For this review, take the finished solid that the model builds, in its own axes (mm). A direction names the side the tool comes from. Round coordinates to 2 decimals unless told otherwise and drop trailing zeros. Write each loop counter-clockwise with the first axis right and the second up, starting at its lowest first coordinate (ties: lowest second). Pieces come first, ordered by that corner, then holes. Notation, with made-up numbers: M 84,53 L 115,53 A12 cw 115,62 Z; hole C 25.5,59 d1. An arc over 180 degrees is marked long. Use one line per item in the form item = value. Start each with the question number.
Item 1: Add section C-C (z = 26). State the section outline as (x, y) points.
Item 2: Draft analysis for pull direction X (two halves, no side actions). For faces 1 (the flat face through (-10, 0, 25)), 2 (the flat face through (19.233, -17, 25)), 3 (the flat face through (-5, -92, 25)), state which applies: released by +X, released by -X, zero draft, split by the parting line, or undercut.
Item 3: Add section D-D (x = -22). State the section outline as (y, z) points, and give its area (3 significant figures).
Item 4: Add section B-B (x = 11). State the section outline as (y, z) points.
Item 5: Add section A-A (y = -18). State the section outline as (x, z) points, and give its area (3 significant figures).
Item 6: For P1, Ø2, axis at y = -21, z = 35, coming from the -X side; P2, Ø10, axis at y = -53.5, z = 5, coming from the +X side; P3, Ø4.5, axis at x = 31, y = -69, coming from the +Z side, all flat-tipped, find the tip position at first contact; note any pin that passes through.
Item 7: For faces 4 (the cylindrical face through (13.724, -86.113, 27.185)), 5 (the flat face through (5, -92, 25)), 6 (the flat face through (-5, -10, 25)), 7 (the flat face through (-19.233, -16, 25)), 8 (the flat face through (7, -93, 27)), list the 3-axis set-ups (+Z, -Z, +X, -X, +Y, -Y) from which the entire face can be reached by the end or side of a thin tool; tool diameter is ignored.
Item 8: For line 1 (X direction, y = -8, z = 37); line 2 (Y direction, x = 0, z = 28); line 3 (X direction, y = -20.5, z = 43.5), list the stretches that pass through material, from the lowest coordinate up. Write a range as [from, to].
from build123d import *

# Parameters (mm, degrees)
F1_DEPTH = 50
F2_DEPTH = 5


# Not quite as in the source:
# - a feature of the source that left no trace in its solid (it failed there, or was rolled back) is left out


with BuildPart() as f1:
    # F0 (on Top) → F1 (new body)
    with BuildSketch(Plane.XY):
        with BuildLine():
            Line((-19.2333690145, -5), (-19.2333690145, -27.8079588042))
            ThreePointArc((-19.2333690145, -27.8079588042), (-36.7344496958, -67.5385811362), (-5, -97.1651718683))
            Line((-5, -97.1651718683), (-5, -87.041634566))
            ThreePointArc((-5, -87.041634566), (-17.5890590993, -38.8605818434), (27.5, -60))
            ThreePointArc((27.5, -60), (25.4982682633, -70.2999182314), (19.7844861402, -79.1003693203))
            ThreePointArc((19.7844861402, -79.1003693203), (13.0128248945, -84.2263573049), (5, -87.041634566))
            Line((5, -87.041634566), (5, -97.1651718683))
            ThreePointArc((5, -97.1651718683), (6.0021906226, -97.0165328972), (7, -96.8408740396))
            Line((7, -96.8408740396), (7, -88.6574597618))
            ThreePointArc((7, -88.6574597618), (13.8146262679, -86.0654196413), (19.7854086015, -81.8812158362))
            Line((19.7854086015, -81.8812158362), (25.5513297312, -87.4477603634))
            ThreePointArc((25.5513297312, -87.4477603634), (26.9788447366, -86.045958164), (28.3295652687, -84.5700169249))
            Line((28.3295652687, -84.5700169249), (22.563644139, -79.0034723976))
            ThreePointArc((22.563644139, -79.0034723976), (27.3526877734, -71.0490031936), (29.4321253055, -62))
            Line((29.4321253055, -62), (37.4466286867, -62))
            ThreePointArc((37.4466286867, -62), (37.4866547971, -61.0003559988), (37.5, -60))
            ThreePointArc((37.5, -60), (32.6151907709, -41.4932625517), (19.2333690145, -27.8079588042))
            Line((19.2333690145, -27.8079588042), (19.2333690145, -5))
            ThreePointArc((19.2333690145, -5), (17.7689029204, -1.4644660941), (14.2333690145, 0))
            Line((14.2333690145, 0), (5, 0))
            Line((5, 0), (5, -20))
            Line((5, -20), (0, -20))
            Line((0, -20), (-5, -20))
            Line((-5, -20), (-5, 0))
            Line((-5, 0), (-14.2333690145, 0))
            ThreePointArc((-14.2333690145, 0), (-17.7689029204, -1.4644660941), (-19.2333690145, -5))
        make_face()
    extrude(amount=F1_DEPTH)

    # F0 (on Top) → F2 (join)
    with BuildSketch(Plane.XY):
        with BuildLine():
            Line((7, -88.6574597618), (7, -96.8408740396))
            ThreePointArc((7, -96.8408740396), (16.9397435916, -93.4558677522), (25.5513297312, -87.4477603634))
            Line((25.5513297312, -87.4477603634), (19.7854086015, -81.8812158362))
            ThreePointArc((19.7854086015, -81.8812158362), (13.8146262679, -86.0654196413), (7, -88.6574597618))
        make_face()
        with BuildLine():
            Line((22.563644139, -79.0034723976), (28.3295652687, -84.5700169249))
            ThreePointArc((28.3295652687, -84.5700169249), (34.7703658136, -74.0453430428), (37.4466286867, -62))
            Line((37.4466286867, -62), (29.4321253055, -62))
            ThreePointArc((29.4321253055, -62), (27.3526877734, -71.0490031936), (22.563644139, -79.0034723976))
        make_face()
    extrude(amount=F2_DEPTH)


solid = f1.part
Calculated:
q1.outline = M -19.23,-27.81 A37.5 ccw -5,-97.17 L -5,-87.04 A27.5 cw long 5,-87.04 L 5,-97.17 A37.5 ccw 7,-96.84 L 7,-88.66 A29.5 ccw 19.79,-81.88 L 25.55,-87.45 A37.5 ccw 28.33,-84.57 L 22.56,-79 A29.5 ccw 29.43,-62 L 37.45,-62 A37.5 ccw 19.23,-27.81 L 19.23,-5 A5 ccw 14.23,0 L 5,0 L 5,-20 L -5,-20 L -5,0 L -14.23,0 A5 ccw -19.23,-5 Z
q2.face_1 = zero draft
q2.face_2 = released by +X
q2.face_3 = undercut
q3.outline = M -90.37,0 L -76.5,0 L -76.5,50 L -90.37,50 Z; M -43.5,0 L -29.63,0 L -29.63,50 L -43.5,50 Z
q3.area = 1,390 mm^2
q4.outline = M -95.85,0 L -85.2,0 L -85.2,50 L -87.37,50 L -87.37,5 L -95.85,5 Z; M -34.8,0 L 0,0 L 0,50 L -34.8,50 Z
q5.outline = M -19.23,0 L -5,0 L -5,50 L -19.23,50 Z; M 5,0 L 19.23,0 L 19.23,50 L 5,50 Z
q5.area = 1,420 mm^2
q6.P1 = -19.23
q6.P2 = 37.47
q6.P3 = 5
q7.face_4 = +Z, -Y
q7.face_5 = +Z, -Z, -Y
q7.face_6 = +Z, -Z, +Y
q7.face_7 = +Z, -Z, -X, +Y
q7.face_8 = +Z, +X, -Y
q8.line_1 = [-19.23, -5], [5, 19.23]
q8.line_2 = [-32.5, -20]
q8.line_3 = [-19.23, 19.23]
